from build123d import *

# Parameters (mm, degrees)
SKETCH1_W           = 20
SKETCH1_H           = 35
BOSS_EXTRUDE1_DEPTH = 7.5
SKETCH3_R           = 4.2
CUT_EXTRUDE1_DEPTH  = 8.5
SKETCH5_R           = 2.5
CUT_EXTRUDE2_DEPTH  = 8.5
SKETCH6_R           = 4
CUT_EXTRUDE3_DEPTH  = 5


with BuildPart() as part:
    # Sketch1 → Boss-Extrude1 (new body)
    with BuildSketch(Plane(origin=(0, 0, 0), x_dir=(1, 0, 0), z_dir=(0, 1, 0))):
        Rectangle(SKETCH1_W, SKETCH1_H)
    extrude(amount=BOSS_EXTRUDE1_DEPTH)

    # Sketch3 → Cut-Extrude1 (cut, through all)
    with BuildSketch(Plane.XZ):
        Circle(SKETCH3_R)
    extrude(amount=-CUT_EXTRUDE1_DEPTH, mode=Mode.SUBTRACT)

    # Sketch5 → Cut-Extrude2 (cut, through all)
    with BuildSketch(Plane.XZ):
        with Locations((0, 10)):
            Circle(SKETCH5_R)
        with Locations((0, -10)):
            Circle(SKETCH5_R)
    extrude(amount=-CUT_EXTRUDE2_DEPTH, mode=Mode.SUBTRACT)

    # Sketch6 → Cut-Extrude3 (cut)
    with BuildSketch(Plane(origin=(0, 7.5, 0), x_dir=(1, 0, 0), z_dir=(0, 1, 0))):
        with Locations((0, 10)):
            Circle(SKETCH6_R)
        with Locations((0, -10)):
            Circle(SKETCH6_R)
    extrude(amount=-CUT_EXTRUDE3_DEPTH, mode=Mode.SUBTRACT)


solid = part.part
The model under review builds one solid part; all positions refer to its coordinate system, in mm. A direction names the side the tool comes from. Round coordinates to 2 decimals unless told otherwise and drop trailing zeros. Write each loop counter-clockwise with the first axis right and the second up, starting at its lowest first coordinate (ties: lowest second). Pieces come first, ordered by that corner, then holes. Notation, with made-up numbers: (64.5, 89) - (95.5, 89) arc R12 cw to (95.5, 106) - close; hole circle Ø9 at (86.25, 65). An arc over 180 degrees is marked (long way). One line per item, written item: value. Start each with the question number.
1. To check wall thickness, follow L1, parallel to Z at x = 0, y = 5.6; L2, parallel to Z at x = 0, y = 1.15; L3, parallel to X at y = 5.2, z = -10. State the ranges of each line that lie inside material, in increasing order. Write a range as from..to.
2. Consider section B-B on y = 6.25. Write out the cut boundary in (x, z), and give its area (3 significant figures).
3. Consider section C-C on x = 0. Write out the cut boundary in (y, z), and give its area (3 significant figures).
4. Clearance check with flat-ended pins moving along their axes: P1, Ø8, axis at x = -0.5, z = 13.5, coming from the +Y side; P2, Ø6, axis at x = 0, z = 10, coming from the +Y side; P3, Ø4.5, axis at x = 0, z = -10, coming from the -Y side. State where each tip first meets the part, or that it passes through.
5. Consider section A-A on z = 0. Write out the cut boundary in (x, y).
6. Consider section D-D on z = 10. Write out the cut boundary in (x, y), and give its area (3 significant figures).
7. The part is to be moulded in two halves that separate along X. For faces 1 (the face through (-2, 7.5, -4)), 2 (the face through (-2, 2.5, -8)), 3 (the face through (-10, 4, 0)), say which applies: released by +X, released by -X, zero draft, split by the parting line, or undercut.
8. Machinability: for faces 4 (the face through (-0.54, 1.23, -12.44)), 5 (the face through (-0.867, 5.035, 13.905)), which of the approach directions +Z, -Z, +X, -X, +Y, -Y give a long, thin tool a straight path to every point of the face, cutting with its end or side? Answer none if there is none.
Checks:
1. L1: z = -17.5..-14, -6..-4.2, 4.2..6, 14..17.5
1. L2: z = -17.5..-12.5, -7.5..-4.2, 4.2..7.5, 12.5..17.5
1. L3: x = -10..-4, 4..10
2. outline: (-10, -17.5) - (10, -17.5) - (10, 17.5) - (-10, 17.5) - close; hole circle Ø8.4 at (0, 0); hole circle Ø8 at (0, -10); hole circle Ø8 at (0, 10)
2. area: 544 mm^2
3. outline: (0, -17.5) - (7.5, -17.5) - (7.5, -14) - (2.5, -14) - (2.5, -12.5) - (0, -12.5) - close; (0, -7.5) - (2.5, -7.5) - (2.5, -6) - (7.5, -6) - (7.5, -4.2) - (0, -4.2) - close; (0, 4.2) - (7.5, 4.2) - (7.5, 6) - (2.5, 6) - (2.5, 7.5) - (0, 7.5) - close; (0, 12.5) - (2.5, 12.5) - (2.5, 14) - (7.5, 14) - (7.5, 17.5) - (0, 17.5) - close
3. area: 94.5 mm^2
4. P1: stops at y = 7.5
4. P2: stops at y = 2.5
4. P3: passes through
5. outline: (-10, 0) - (-4.2, 0) - (-4.2, 7.5) - (-10, 7.5) - close; (4.2, 0) - (10, 0) - (10, 7.5) - (4.2, 7.5) - close
6. outline: (-10, 0) - (-2.5, 0) - (-2.5, 2.5) - (-4, 2.5) - (-4, 7.5) - (-10, 7.5) - close; (2.5, 0) - (10, 0) - (10, 7.5) - (4, 7.5) - (4, 2.5) - (2.5, 2.5) - close
6. area: 97.5 mm^2
7. face 1: zero draft
7. face 2: undercut
7. face 3: released by -X
8. face 4: +Y, -Y
8. face 5: +Y
